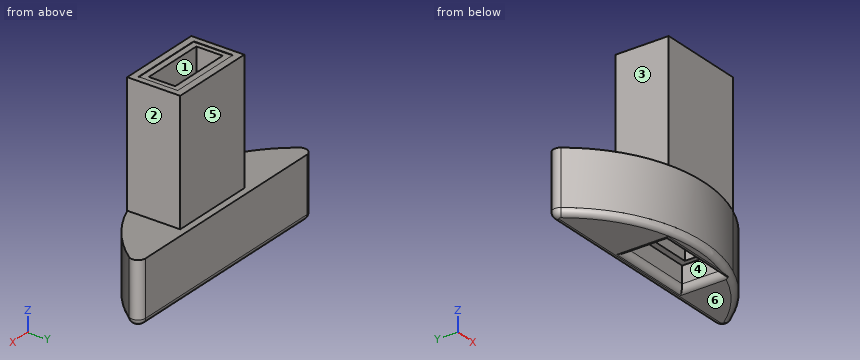
from build123d import *

# Parameters (mm, degrees)
F0_W         = 1.275
F0_H         = 0.8956698048
F0_H_2       = 0.9093301952
F0_H_3       = 0.8412417081
F1_DEPTH     = 8
F2_DEPTH     = 3
F3_DEPTH     = 21
F4_DEPTH     = 24.05
F5_R         = 1
F6_T1_DEPTH  = 28.6496073272
F6_T3_DEPTH  = 9.8
F6_T5_DEPTH  = 5.15
F6_T8_ANGLE  = 126.6295364974
F6_T10_ANGLE = 126.6295364974
F6_T12_ANGLE = 106.7409270051
F6_T17_DEPTH = 11.8
F6_T21_DEPTH = 7.15
F6_T28_DEPTH = 11.8
F6_T32_DEPTH = 7.15
F6_T39_DEPTH = 7.15
F6_T43_DEPTH = 11.8
F6_T50_DEPTH = 11.8
F6_T54_DEPTH = 7.15


# Not quite as in the source:
# - a fillet or chamfer that OpenCascade refuses, or shapes differently, is made with other operations: its cross-section is extruded or revolved along the edge and cut away or added


with BuildPart() as f1:
    # F0 (on Top) → F1 (new body)
    with BuildSketch(Plane.XY):
        with BuildLine():
            Line((0, -9.65), (-16.1925908983, -9.65))
            ThreePointArc((-16.1925908983, -9.65), (-6.0604727533, -17.8491784127), (6.9692709671, -17.5143301952))
            Line((6.9692709671, -17.5143301952), (-4.4192709671, -17.5143301952))
            Line((-4.4192709671, -17.5143301952), (-4.4192709671, -10.5456698048))
            Line((-4.4192709671, -10.5456698048), (0, -10.5456698048))
            Line((0, -10.5456698048), (0, -9.65))
        make_face()
        with BuildLine():
            ThreePointArc((6.9692709671, -17.5143301952), (12.2302855086, -14.3437309086), (16.1925908983, -9.65))
            Line((16.1925908983, -9.65), (1.275, -9.65))
            Line((1.275, -9.65), (1.275, -10.5456698048))
            Line((1.275, -10.5456698048), (6.9692709671, -10.5456698048))
            Line((6.9692709671, -10.5456698048), (6.9692709671, -17.5143301952))
        make_face()
        with Locations((0.6375, -10.0978349024)):
            Rectangle(F0_W, F0_H)
        Polygon((-4.4192709671, -17.5143301952), (6.9692709671, -17.5143301952), (6.9692709671, -10.5456698048), (1.275, -10.5456698048), (1.275, -11.455), (6.175, -11.455), (6.175, -16.605), (-3.625, -16.605), (-3.625, -11.455), (0, -11.455), (0, -10.5456698048), (-4.4192709671, -10.5456698048), align=None)
        with Locations((0.6375, -11.0003349024)):
            Rectangle(F0_W, F0_H_2)
        Polygon((0, -12.2962417081), (0, -11.455), (-3.625, -11.455), (-3.625, -16.605), (6.175, -16.605), (6.175, -11.455), (1.275, -11.455), (1.275, -12.2962417081), (5.4913964123, -12.2962417081), (5.4913964123, -15.7637582919), (-2.9413964123, -15.7637582919), (-2.9413964123, -12.2962417081), align=None)
        with Locations((0.6375, -11.875620854)):
            Rectangle(F0_W, F0_H_3)
    extrude(amount=F1_DEPTH)

    # F0 (on Top) → F2 (cut)
    with BuildSketch(Plane.XY):
        Polygon((0, -12.2962417081), (0, -11.455), (-3.625, -11.455), (-3.625, -16.605), (6.175, -16.605), (6.175, -11.455), (1.275, -11.455), (1.275, -12.2962417081), (5.4913964123, -12.2962417081), (5.4913964123, -15.7637582919), (-2.9413964123, -15.7637582919), (-2.9413964123, -12.2962417081), align=None)
        with Locations((0.6375, -11.875620854)):
            Rectangle(F0_W, F0_H_3)
    extrude(amount=F2_DEPTH, mode=Mode.SUBTRACT)

    # F3 (add): a face of the model
    f3_faces = [f1.faces().sort_by_distance(p)[0] for p in [
        (1.275, -16.4942920509, 3),
    ]]
    extrude(f3_faces, amount=-F3_DEPTH)

    # F0 (on Top) → F4 (join)
    with BuildSketch(Plane.XY):
        Polygon((-4.4192709671, -17.5143301952), (6.9692709671, -17.5143301952), (6.9692709671, -10.5456698048), (1.275, -10.5456698048), (1.275, -11.455), (6.175, -11.455), (6.175, -16.605), (-3.625, -16.605), (-3.625, -11.455), (0, -11.455), (0, -10.5456698048), (-4.4192709671, -10.5456698048), align=None)
        with Locations((0.6375, -11.0003349024)):
            Rectangle(F0_W, F0_H_2)
    extrude(amount=F4_DEPTH)

    # F5
    f5_edges = [f1.edges().sort_by_distance(p)[0] for p in [
        (16.192591, -9.65, 4),
        (-16.192591, -9.65, 4),
    ]]
    fillet(f5_edges, radius=F5_R)

    # F6: fillet of radius 0.8 on 8 edges, made by hand

    # F6_s2 → F6_t1 (cut)
    with BuildSketch(Plane.YZ.offset(-14.3248036636)):
        with BuildLine():
            ThreePointArc((-10.45, 0), (-9.8843145751, 0.2343145751), (-9.65, 0.8))
            Line((-9.65, 0.8), (-9.65, 0))
            Line((-9.65, 0), (-10.45, 0))
        make_face()
    extrude(amount=F6_T1_DEPTH, mode=Mode.SUBTRACT)

    # F6_s4 → F6_t3 (cut)
    with BuildSketch(Plane.YZ.offset(-3.625)):
        with BuildLine():
            ThreePointArc((-17.405, 0), (-16.8393145751, 0.2343145751), (-16.605, 0.8))
            Line((-16.605, 0.8), (-16.605, 0))
            Line((-16.605, 0), (-17.405, 0))
        make_face()
        with BuildLine():
            ThreePointArc((-10.655, 0), (-11.2206854249, 0.2343145751), (-11.455, 0.8))
            Line((-11.455, 0.8), (-11.455, 0))
            Line((-11.455, 0), (-10.655, 0))
        make_face()
    extrude(amount=F6_T3_DEPTH, mode=Mode.SUBTRACT)

    # F6_s6 → F6_t5 (cut)
    with BuildSketch(Plane.XZ.offset(11.455)):
        with BuildLine():
            ThreePointArc((-4.425, 0), (-3.8593145751, 0.2343145751), (-3.625, 0.8))
            Line((-3.625, 0.8), (-3.625, 0))
            Line((-3.625, 0), (-4.425, 0))
        make_face()
        with BuildLine():
            ThreePointArc((6.975, 0), (6.4093145751, 0.2343145751), (6.175, 0.8))
            Line((6.175, 0.8), (6.175, 0))
            Line((6.175, 0), (6.975, 0))
        make_face()
    extrude(amount=F6_T5_DEPTH, mode=Mode.SUBTRACT)

    # F6_s7 → F6_t8 (revolve, cut)
    with BuildSketch(Plane(origin=(0, 0, 0), x_dir=(0, 0, 1), z_dir=(-0.5966386555, -0.8025100092, 0))):
        with BuildLine():
            ThreePointArc((0, -18.05), (0.2343145751, -18.6156854249), (0.8, -18.85))
            Line((0.8, -18.85), (0, -18.85))
            Line((0, -18.85), (0, -18.05))
        make_face()
    revolve(axis=Axis((14.3248036636, -10.65, 0), (0, 0, 1)), revolution_arc=F6_T8_ANGLE, mode=Mode.SUBTRACT)

    # F6_s9 → F6_t10 (revolve, cut)
    with BuildSketch(Plane(origin=(0, 0, 0), x_dir=(0, 0, 1), z_dir=(0.5966386555, -0.8025100092, 0))):
        with BuildLine():
            ThreePointArc((0, 18.05), (0.2343145751, 18.6156854249), (0.8, 18.85))
            Line((0.8, 18.85), (0, 18.85))
            Line((0, 18.85), (0, 18.05))
        make_face()
    revolve(axis=Axis((-14.3248036636, -10.65, 0), (0, 0, -1)), revolution_arc=F6_T10_ANGLE, mode=Mode.SUBTRACT)

    # F6_s11 → F6_t12 (revolve, cut)
    with BuildSketch(Plane(origin=(0, 0, 0), x_dir=(0, 0, 1), z_dir=(-0.5966386555, 0.8025100092, 0))):
        with BuildLine():
            ThreePointArc((0.8, -18.85), (0.2343145751, -18.6156854249), (0, -18.05))
            Line((0, -18.05), (0, -18.85))
            Line((0, -18.85), (0.8, -18.85))
        make_face()
    revolve(axis=Axis((0, 0, 0), (0, 0, 1)), revolution_arc=F6_T12_ANGLE, mode=Mode.SUBTRACT)


with BuildPart() as f6_tool15:
    # F6_s16 → F6_t17 (new body)
    with BuildSketch(Plane.YZ.offset(-5.625)):
        with BuildLine():
            ThreePointArc((-17.405, 0), (-16.8393145751, 0.2343145751), (-16.605, 0.8))
            Line((-16.605, 0.8), (-16.605, 0))
            Line((-16.605, 0), (-17.405, 0))
        make_face()
    extrude(amount=F6_T17_DEPTH)

    split(bisect_by=Plane.YZ.offset(-3.625), keep=Keep.BOTTOM)


with BuildPart() as f6_tool19:
    # F6_s20 → F6_t21 (new body)
    with BuildSketch(Plane.XZ.offset(11.455)):
        with BuildLine():
            ThreePointArc((-4.425, 0), (-3.8593145751, 0.2343145751), (-3.625, 0.8))
            Line((-3.625, 0.8), (-3.625, 0))
            Line((-3.625, 0), (-4.425, 0))
        make_face()
    extrude(amount=F6_T21_DEPTH)

    split(bisect_by=Plane.XZ.offset(16.605), keep=Keep.TOP)


with BuildPart() as f6_tool15_1:
    add(f6_tool15.part)

    # F6_t23: intersect F6_tool19
    add(f6_tool19.part, mode=Mode.INTERSECT)


with BuildPart() as f1_1:
    add(f1.part)

    # F6_t13: cut F6_tool15
    add(f6_tool15_1.part, mode=Mode.SUBTRACT)


with BuildPart() as f6_tool26:
    # F6_s27 → F6_t28 (new body)
    with BuildSketch(Plane.YZ.offset(-3.625)):
        with BuildLine():
            ThreePointArc((-17.405, 0), (-16.8393145751, 0.2343145751), (-16.605, 0.8))
            Line((-16.605, 0.8), (-16.605, 0))
            Line((-16.605, 0), (-17.405, 0))
        make_face()
    extrude(amount=F6_T28_DEPTH)

    split(bisect_by=Plane.YZ.offset(6.175), keep=Keep.TOP)


with BuildPart() as f6_tool30:
    # F6_s31 → F6_t32 (new body)
    with BuildSketch(Plane.XZ.offset(18.605)):
        with BuildLine():
            ThreePointArc((6.975, 0), (6.4093145751, 0.2343145751), (6.175, 0.8))
            Line((6.175, 0.8), (6.175, 0))
            Line((6.175, 0), (6.975, 0))
        make_face()
    extrude(amount=-F6_T32_DEPTH)

    split(bisect_by=Plane.XZ.offset(16.605), keep=Keep.TOP)


with BuildPart() as f6_tool26_1:
    add(f6_tool26.part)

    # F6_t34: intersect F6_tool30
    add(f6_tool30.part, mode=Mode.INTERSECT)


with BuildPart() as f1_2:
    add(f1_1.part)

    # F6_t24: cut F6_tool26
    add(f6_tool26_1.part, mode=Mode.SUBTRACT)


with BuildPart() as f6_tool37:
    # F6_s38 → F6_t39 (new body)
    with BuildSketch(Plane.XZ.offset(9.455)):
        with BuildLine():
            ThreePointArc((-4.425, 0), (-3.8593145751, 0.2343145751), (-3.625, 0.8))
            Line((-3.625, 0.8), (-3.625, 0))
            Line((-3.625, 0), (-4.425, 0))
        make_face()
    extrude(amount=F6_T39_DEPTH)

    split(bisect_by=Plane.XZ.offset(11.455), keep=Keep.BOTTOM)


with BuildPart() as f6_tool41:
    # F6_s42 → F6_t43 (new body)
    with BuildSketch(Plane.YZ.offset(6.175)):
        with BuildLine():
            ThreePointArc((-10.655, 0), (-11.2206854249, 0.2343145751), (-11.455, 0.8))
            Line((-11.455, 0.8), (-11.455, 0))
            Line((-11.455, 0), (-10.655, 0))
        make_face()
    extrude(amount=-F6_T43_DEPTH)

    split(bisect_by=Plane.YZ.offset(-3.625), keep=Keep.BOTTOM)


with BuildPart() as f6_tool37_1:
    add(f6_tool37.part)

    # F6_t45: intersect F6_tool41
    add(f6_tool41.part, mode=Mode.INTERSECT)


with BuildPart() as f1_3:
    add(f1_2.part)

    # F6_t35: cut F6_tool37
    add(f6_tool37_1.part, mode=Mode.SUBTRACT)


with BuildPart() as f6_tool48:
    # F6_s49 → F6_t50 (new body)
    with BuildSketch(Plane.YZ.offset(8.175)):
        with BuildLine():
            ThreePointArc((-10.655, 0), (-11.2206854249, 0.2343145751), (-11.455, 0.8))
            Line((-11.455, 0.8), (-11.455, 0))
            Line((-11.455, 0), (-10.655, 0))
        make_face()
    extrude(amount=-F6_T50_DEPTH)

    split(bisect_by=Plane.YZ.offset(6.175), keep=Keep.TOP)


with BuildPart() as f6_tool52:
    # F6_s53 → F6_t54 (new body)
    with BuildSketch(Plane.XZ.offset(16.605)):
        with BuildLine():
            ThreePointArc((6.975, 0), (6.4093145751, 0.2343145751), (6.175, 0.8))
            Line((6.175, 0.8), (6.175, 0))
            Line((6.175, 0), (6.975, 0))
        make_face()
    extrude(amount=-F6_T54_DEPTH)

    split(bisect_by=Plane.XZ.offset(11.455), keep=Keep.BOTTOM)


with BuildPart() as f6_tool48_1:
    add(f6_tool48.part)

    # F6_t56: intersect F6_tool52
    add(f6_tool52.part, mode=Mode.INTERSECT)


with BuildPart() as f1_4:
    add(f1_3.part)

    # F6_t46: cut F6_tool48
    add(f6_tool48_1.part, mode=Mode.SUBTRACT)


solid = f1_4.part
The model under review builds one solid part; all positions refer to its coordinate system, in mm. Face numbers are marked on the shaded views. A direction names the side the tool comes from. Round coordinates to 2 decimals unless told otherwise and drop trailing zeros. Loops run counter-clockwise (first coordinate to the right, second up) from the corner with the lowest first, then second, coordinate; pieces in that order, holes last. Notation, with made-up numbers: (35, 45.5) - (75, 45.5) arc R20 cw to (75, 63.5) - close; hole circle Ø11 at (-0.5, 45.5). An arc over 180 degrees is marked (long way). Use CSV: the item, a comma, the result in double quotes.
(1) Take a section at A-A, the plane z = 20.5. Give the boundary of the cut face in (x, y), plus the area to 3 significant figures.
Working result:
outline,"(-4.42, -17.51) - (6.97, -17.51) - (6.97, -10.55) - (-4.42, -10.55) - close; hole (-2.94, -15.76) - (5.49, -15.76) - (5.49, -12.3) - (-2.94, -12.3) - close"
area,"50.1 mm^2"
(2) Clearance check with flat-ended pins moving along their axes: P1, Ø12.5, axis at x = 3.5, z = 18.5, coming from the -Y side; P2, Ø2, axis at y = -17, z = 11, coming from the -X side; P3, Ø9, axis at x = 1.5, z = 19, coming from the +Y side. State where each tip first meets the part, or that it passes through.
Working result:
P1,"stops at y = -17.51"
P2,"stops at x = -4.42"
P3,"stops at y = -10.55"
(3) The part is to be moulded in two halves that separate along Y. For the marked faces 4, 5 and 6, say which applies: pulls with the +Y half, pulls with the -Y half, needs draft (parallel to the pull), parting line crosses it, or undercut.
Working result:
face 4,"undercut"
face 5,"pulls with the +Y half"
face 6,"needs draft"
(4) For line 1 (X direction, y = -13.5, z = 15.5); line 2 (Y direction, x = -0.5, z = 9); line 3 (X direction, y = -11.5, z = 22.25), list the stretches that pass through material, from the lowest coordinate up.
Working result:
line 1,"x = -4.42 to -2.94, 5.49 to 6.97"
line 2,"y = -17.51 to -15.76, -12.3 to -10.55"
line 3,"x = -4.42 to 6.97"
(5) Machinability: for the marked faces 1, 2 and 3, which of the approach directions +Z, -Z, +X, -X, +Y, -Y give a long, thin tool a straight path to every point of the face, cutting with its end or side? Answer none if there is none.
Working result:
face 1,"+Z, -Z"
face 2,"+Z, +X, +Y, -Y"
face 3,"+Z, -X, +Y, -Y"
